```python
from build123d import *

# Parameters (mm, degrees)
P_IDAT_VYSUNUT_M1_DEPTH  = 3
P_IDAT_VYSUNUT_M2_DEPTH  = 2
ZAOBLIT4_R               = 1
SKICA2_W                 = 4
SKICA2_H                 = 2
ODEBRAT_VYSUNUT_M2_DEPTH = 0.8
SKICA3_W                 = 4
SKICA3_H                 = 2
ODEBRAT_VYSUNUT_M3_DEPTH = 0.8


with BuildPart() as part:
    # Skica1 → P_idat vysunut_m1 (new body)
    with BuildSketch(Plane(origin=(0, 0, 0), x_dir=(1, 0, 0), z_dir=(0, 1, 0))):
        Polygon((-118.143750166, 15), (-118.143750166, 0), (-68.779346971, 32.313398106), (-16.32734533, 12.51119421), (-26.593132493, 30.830954414), (-20.343228113, 42.230019956), (0, 37.22), (0, 69.22), (-39.317553332, 46.52), (-78.635106664, 69.22), (-118.143185584, 46.41), (-118.143185584, 33.5570142), (-107.643750166, 37.378496169), (-107.643750166, 24.278496169), (-128.093750166, 24.278496169), (-128.093750166, 11.378496169), align=None)
    extrude(amount=P_IDAT_VYSUNUT_M1_DEPTH)

    # Skica1_5 → P_idat vysunut_m2 (add)
    with BuildSketch(Plane(origin=(0, 0, 0), x_dir=(1, 0, 0), z_dir=(0, 1, 0))):
        Polygon((-68.779346971, 32.313398106), (-118.143750166, 0), (0, 0), (0, 15), (9.950504516, 11.37831254), (9.950504516, 24.27831254), (-10.5, 24.27831254), (-10.5, 37.37831254), (0, 33.55662508), (0, 37.22), (-20.343228113, 42.230019956), (-26.593132493, 30.830954414), (-16.32734533, 12.51119421), align=None)
    extrude(amount=P_IDAT_VYSUNUT_M2_DEPTH)

    # Zaoblit4
    zaoblit4_edges = [part.edges().sort_by_distance(p)[0] for p in [
        (-118.143750166, 1.5, -15),
        (-128.093750166, 1.5, -11.378496169),
        (-128.093750166, 1.5, -24.278496169),
        (-107.643750166, 1.5, -24.278496169),
        (-107.643750166, 1.5, -37.378496169),
        (-118.143185584, 1.5, -33.5570142),
        (-10.5, 1, -24.27831254),
        (-10.5, 1, -37.37831254),
        (0, 1, -33.55662508),
        (0, 1, -15),
        (9.950504516, 1, -11.37831254),
        (9.950504516, 1, -24.27831254),
    ]]
    fillet(zaoblit4_edges, radius=ZAOBLIT4_R)

    # Skica2 → Odebrat vysunut_m2 (cut)
    with BuildSketch(Plane(origin=(0, 3, 0), x_dir=(1, 0, 0), z_dir=(0, 1, 0))):
        with Locations((-126.093750166, 20.342570172)):
            Rectangle(SKICA2_W, SKICA2_H)
    extrude(amount=-ODEBRAT_VYSUNUT_M2_DEPTH, mode=Mode.SUBTRACT)

    # Skica3 → Odebrat vysunut_m3 (cut)
    with BuildSketch(Plane(origin=(0, 2, 0), x_dir=(1, 0, 0), z_dir=(0, 1, 0))):
        with Locations((-12.5, 32.914238537)):
            Rectangle(SKICA3_W, SKICA3_H)
    extrude(amount=-ODEBRAT_VYSUNUT_M3_DEPTH, mode=Mode.SUBTRACT)


solid = part.part
```
Work out the finished part from the listing and answer in its coordinate system (mm). A direction names the side the tool comes from. Coordinates: 2 decimals unless noted, no trailing zeros. Write each loop counter-clockwise with the first axis right and the second up, starting at its lowest first coordinate (ties: lowest second). Pieces come first, ordered by that corner, then holes.
Q1. A cutting plane is placed at C-C, the plane z = -29. Give the vertices of the cut face in (x, y).
Q2. A cutting plane is placed at D-D, the plane x = -44.5. Give the vertices of the cut face in (y, z), then the cut area to 3 significant figures.
Q3. Determine the mould class of faces 1 (the face through (-112.948, 1.479, -35.448)), 2 (the face through (0, 1, -52)), 3 (the face through (-118.143, 1, -41)), 4 (the face through (-65, 3, -43)) for opening direction X: released by +X, released by -X, zero draft, split by the parting line, or undercut.
Q4. Find the intervals of material crossed by line 1 (Y direction, x = -8, z = -13.5); line 2 (X direction, y = 0.4, z = -3); line 3 (Z direction, x = -21, y = 2.6), in increasing order.
Q5. Which of the six approach directions +Z, -Z, +X, -X, +Y, -Y give full straight-line access (tool end or side, diameter ignored) to faces 5 (the face through (-5.305, 0.986, -35.487)), 6 (the face through (-21.388, 2.493, -21.543)), 7 (the face through (-10.31, 2.49, -39.76))?
Q6. A cutting plane is placed at B-B, the plane x = -114.5. Give the vertices of the cut face in (y, z).
Q7. Each of these flat-tipped pins is pushed along its axis until it touches: pin 1 Ø0.9 at (x, y) = (-126, 2.5) entering from -Z; pin 2 Ø1.6 at (y, z) = (0.5, -31) entering from +X; pin 3 Ø12.5 at (x, z) = (-76, -13.5) entering from +Y. Where does it stop, or does it pass through?
Findings below:
1. outline: (-107.64, 0) - (-10.5, 0) - (-10.5, 2) - (-25.57, 2) - (-25.57, 3) - (-60, 3) - (-60, 2) - (-73.84, 2) - (-73.84, 3) - (-107.64, 3) - close
2. outline: (0, -49.51) - (3, -49.51) - (3, -23.15) - (2, -23.15) - (2, 0) - (0, 0) - close
2. area: 125 mm2
3. face 1: undercut
3. face 2: released by +X
3. face 3: released by -X
3. face 4: zero draft
4. line 1: y = 0 to 2
4. line 2: x = -118.14 to 0
4. line 3: z = -57.1 to -41.03, -20.85 to -14.28
5. face 5: +Y, -Y
5. face 6: +X, +Y
5. face 7: +Y
6. outline: (0, -48.51) - (3, -48.51) - (3, -34.88) - (0, -34.88) - close; (0, -24.28) - (3, -24.28) - (3, -2.39) - (2, -2.39) - (2, 0) - (0, 0) - close
7. pin 1: stops at z = -24.28
7. pin 2: stops at x = -10.5
7. pin 3: stops at y = 2
